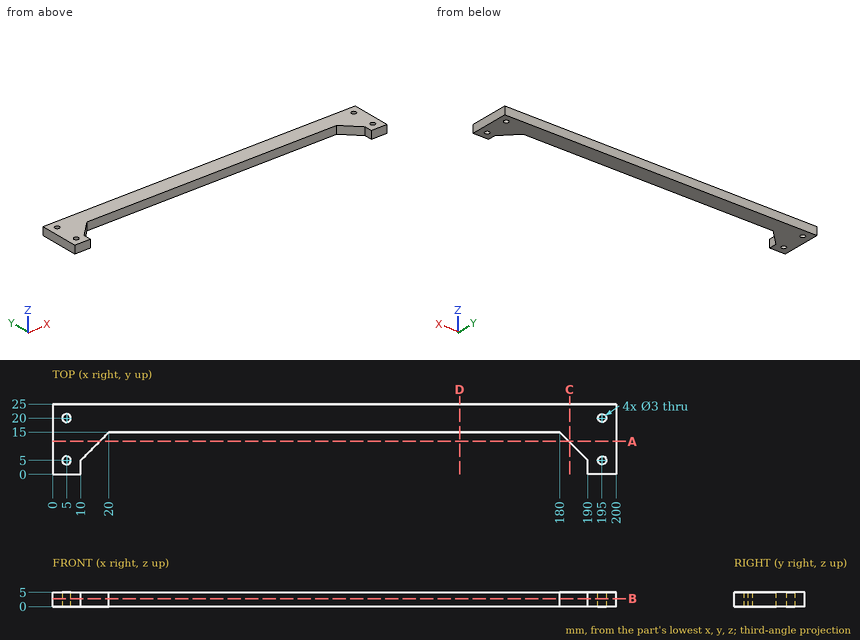
Here's the drawing with two shaded views (mm, measured from the low corner). I have some questions. Coordinates: 2 decimals unless noted, no trailing zeros. Write each loop counter-clockwise with the first axis right and the second up, starting at its lowest first coordinate (ties: lowest second). Pieces come first, ordered by that corner, then holes. Notation, with made-up numbers: M 3,-30.75 L 14,-30.75 A25 cw 14,8.25 Z; hole C 32,-1 d9. An arc over 180 degrees is marked long. Write item = value, one per line. Start each with the question number.
Q1. If we section it at A-A, the plane y = 11.75: Write out the boundary of the cut face in (x, z).
Q2. If I drill on L1, parallel to Y at x = 5, z = 2.7; L2, parallel to X at y = 21, z = 4.3; L3, parallel to Y at x = 68, z = 4, over which ranges is the centre line in solid material (lowest first)? Write a range as [from, to].
Q3. If we section it at B-B, the plane z = 2.8: Write out the boundary of the cut face in (x, y).
Q4. I'm going to push a flat-ended pin straight in: pin 1 (2 mm diameter, centred on x = 153, z = 2, fed in from -Y). Where does the tip first touch, or does it pass through?
Q5. If we section it at C-C, the plane x = 183.5: Write out the boundary of the cut face in (y, z).
Q6. If we section it at D-D, the plane x = 144.5: Write out the boundary of the cut face in (y, z), then the cut area to 3 significant figures.
Check sheet entries:
q1.outline = M 0,0 L 16.75,0 L 16.75,5 L 0,5 Z; M 183.25,0 L 200,0 L 200,5 L 183.25,5 Z
q2.L1 = [0, 3.5], [6.5, 18.5], [21.5, 25]
q2.L2 = [0, 3.88], [6.12, 193.88], [196.12, 200]
q2.L3 = [15, 25]
q3.outline = M 0,0 L 10,0 L 10,5 L 20,15 L 180,15 L 190,5 L 190,0 L 200,0 L 200,25 L 0,25 Z; hole C 5,5 d3; hole C 5,20 d3; hole C 195,5 d3; hole C 195,20 d3
q4.pin_1 = 15
q5.outline = M 11.5,0 L 25,0 L 25,5 L 11.5,5 Z
q6.outline = M 15,0 L 25,0 L 25,5 L 15,5 Z
q6.area = 50.0 mm²
